Geometry check sheet. Reference: the model listing, model coordinates, mm. Face numbers are marked on the shaded views. A direction names the side the tool comes from. Coordinates: 2 decimals unless noted, no trailing zeros. Loops run counter-clockwise (first coordinate to the right, second up) from the corner with the lowest first, then second, coordinate; pieces in that order, holes last. Notation, with made-up numbers: (72.25, 76) - (107.25, 76) arc R32 cw to (107.25, 109) - close; hole circle Ø8 at (76.5, -2). An arc over 180 degrees is marked (long way). One line per item, written item: value.
from build123d import *

# Parameters (mm, degrees)
PAD_DEPTH    = 15
POCKET_DEPTH = 13.75


with BuildPart() as part:
    # Sketch → Pad (new body)
    with BuildSketch(Plane.XY):
        with BuildLine():
            Line((-27.52, 9.5), (27.52, 9.5))
            ThreePointArc((30, 7.02), (29.273625, 8.773625), (27.52, 9.5))
            Line((30, 7.02), (30, -7.02))
            ThreePointArc((27.52, -9.5), (29.273625, -8.773625), (30, -7.02))
            Line((27.52, -9.5), (-27.52, -9.5))
            ThreePointArc((-30, -7.02), (-29.273625, -8.773625), (-27.52, -9.5))
            Line((-30, -7.02), (-30, 7.02))
            ThreePointArc((-27.52, 9.5), (-29.273625, 8.773625), (-30, 7.02))
        make_face()
    extrude(amount=PAD_DEPTH)

    # Sketch001 (on Face10 of Pad) → Pocket (cut)
    with BuildSketch(Plane.XY.offset(15)):
        Polygon((-30.255, 2), (-11.625, 2), (-11.625, 4.6), (11.625, 4.6), (11.625, 2), (30.255, 2), (30.255, -2), (11.625, -2), (11.625, -4.6), (-11.625, -4.6), (-11.625, -2), (-30.255, -2), align=None)
    extrude(amount=-POCKET_DEPTH, mode=Mode.SUBTRACT)


solid = part.part
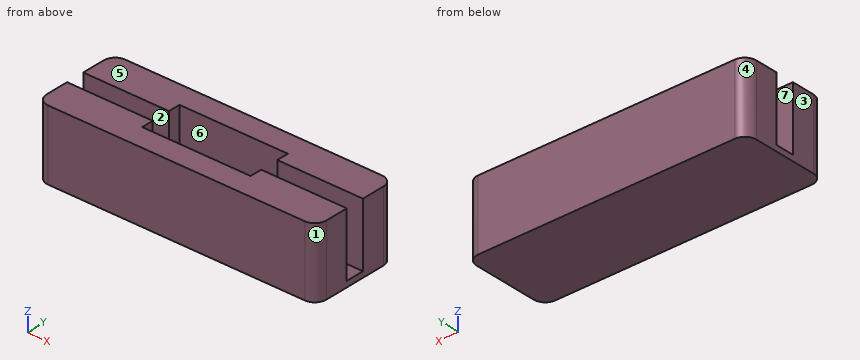
(1) Cross-section at B-B on x = 10.5. Record the cut outline in (y, z).
Reply:
outline: (-9.5, 0) - (9.5, 0) - (9.5, 15) - (4.6, 15) - (4.6, 1.25) - (-4.6, 1.25) - (-4.6, 15) - (-9.5, 15) - close
(2) Cross-section at A-A on z = 5.75. Record the cut outline in (x, y) (3 decimals), and give its area (3 significant figures).
Reply:
outline: (-30, -7.02) arc R2.48 ccw to (-27.52, -9.5) - (27.52, -9.5) arc R2.48 ccw to (30, -7.02) - (30, -2) - (11.625, -2) - (11.625, -4.6) - (-11.625, -4.6) - (-11.625, -2) - (-30, -2) - close; (-30, 2) - (-11.625, 2) - (-11.625, 4.6) - (11.625, 4.6) - (11.625, 2) - (30, 2) - (30, 7.02) arc R2.48 ccw to (27.52, 9.5) - (-27.52, 9.5) arc R2.48 ccw to (-30, 7.02) - close
area: 774 mm2
(3) Access from +Z, -Z, +X, -X, +Y, -Y to the whole of each face (thin tool, end or side, straight path). Record for the marked faces 5, 6 and 7.
Reply:
face 5: +Z, +X, -X, +Y, -Y
face 6: +Z
face 7: +Z, +X, -X
(4) Material ranges on probe 1 along Y at (x, z) = (10.5, 6.5); probe 2 along X at (y, z) = (-2.5, 10.5) (3 decimals); probe 3 along Y at (x, z) = (-22.5, 6.75), recorded low to high. Write a range as from..to.
Reply:
probe 1: -9.5..-4.6, 4.6..9.5
probe 2: -30..-11.625, 11.625..30
probe 3: -9.5..-2, 2..9.5
(5) Cross-section at C-C on y = 3.5. Record the cut outline in (x, z) (3 decimals), and give its area (3 significant figures).
Reply:
outline: (-30, 0) - (30, 0) - (30, 15) - (11.625, 15) - (11.625, 1.25) - (-11.625, 1.25) - (-11.625, 15) - (-30, 15) - close
area: 580 mm2
(6) Release check for a two-part mould opening along Y. For the marked faces 1, 2, 3 and 4 record: pulls with the +Y half, pulls with the -Y half, needs draft (parallel to the pull), parting line crosses it, or undercut.
Reply:
face 1: pulls with the -Y half
face 2: undercut
face 3: needs draft
face 4: pulls with the +Y half
